The model under review builds one solid part; all positions refer to its coordinate system, in mm. A direction names the side the tool comes from. Give positions to 0.01 mm unless a question says otherwise; leave off trailing zeros. Loops run counter-clockwise (first coordinate to the right, second up) from the corner with the lowest first, then second, coordinate; pieces in that order, holes last. Notation, with made-up numbers: M -37,86 L -5,86 A23 ccw -5,112 Z; hole C 1,12 d9. An arc over 180 degrees is marked long. Write item = value, one per line. Start each with the question number.
1. Draft analysis for pull direction Y (two halves, no side actions). For faces 1 (the face through (8.5, 1.11, 43.65)), 2 (the face through (-6.33, 2.36, 43.65)), 3 (the face through (0, -3.969, 23)), state which applies: pulls with the +Y half, pulls with the -Y half, needs draft (parallel to the pull), parting line crosses it, or undercut.
2. We need section D-D on z = 26.5. Give the boundary of the cut face in (x, y) (3 decimals).
3. For faces 4 (the face through (6.236, -2.417, 43.645)), 5 (the face through (-12.687, -0.496, 4.829)), 6 (the face through (-9.181, -0.714, 43.645)), list the 3-axis set-ups (+Z, -Z, +X, -X, +Y, -Y) from which the entire face can be reached by the end or side of a thin tool; tool diameter is ignored.
4. We need section C-C on z = 39.5. Give the boundary of the cut face in (x, y) (3 decimals), then the cut area to 3 significant figures.
5. We need section B-B on x = 1.5. Give the boundary of the cut face in (y, z), then the cut area to 3 significant figures.
6. We need section A-A on z = 10. Give the boundary of the cut face in (x, y) (1 decimal).
7. Wall thickness on line 1 along Y through (x, z) = (11, 4); line 2 along Z through (x, y) = (-8.5, -1.5); line 3 along Z through (x, y) = (5, -1.75): over which ranges is each line inside the solid? List them lowest first. Write a range as from..to.
8. For pin 1 (4 mm diameter, centred on y = -2, z = 33, fed in from +X) (3 decimals); pin 2 (1 mm diameter, centred on x = -6, z = 10.5, fed in from -Y); pin 3 (3 mm diameter, centred on x = 11.11, y = 0, fed in from -Z); pin 4 (2.5 mm diameter, centred on x = 5.5, y = 1, fed in from +Z), all flat-tipped, find the tip position at first contact; note any pin that passes through.
from build123d import *

# Parameters (mm, degrees)
F0_R     = 7.9375
F0_R_2   = 3.175
F1_DEPTH = 3.96875
F2_R     = 0.79375
F4_D     = 3.302
F4_DEPTH = 9.525
F4_TIP   = 0.992020882
F6_R     = 3.302
F7_DEPTH = 25.4
F9_DEPTH = 1.5875


with BuildPart() as f1:
    # F0 (on Front) → F1 (new body, symmetric)
    with BuildSketch(Plane.XZ):
        with BuildLine():
            Line((-15.875, 7.9375), (-15.875, 0))
            Line((-15.875, 0), (15.875, 0))
            Line((15.875, 0), (15.875, 7.9375))
            Line((15.875, 7.9375), (9.525, 25.4))
            Line((9.525, 25.4), (9.525, 42.8625))
            Line((9.525, 42.8625), (5.9398811015, 42.8625))
            ThreePointArc((5.9398811015, 42.8625), (0, 46.0375), (-5.9398811015, 42.8625))
            Line((-5.9398811015, 42.8625), (-9.525, 42.8625))
            Line((-9.525, 42.8625), (-9.525, 25.4))
            Line((-9.525, 25.4), (-15.875, 7.9375))
        make_face()
        with Locations((0, 12.7)):
            Circle(F0_R, mode=Mode.SUBTRACT)
        with Locations((0, 38.89375)):
            Circle(F0_R_2, mode=Mode.SUBTRACT)
    extrude(amount=F1_DEPTH, both=True)

    # F2
    f2_edges = [f1.edges().sort_by_distance(p)[0] for p in [
        (-9.525, 0, 42.8625),
        (9.525, 0, 42.8625),
    ]]
    fillet(f2_edges, radius=F2_R)

    # F4
    with Locations(Plane(origin=(0, 0, 0), x_dir=(1, 0, 0), z_dir=(0, 0, -1))):
        with Locations((-11.1125, 0), (11.1125, 0)):
            Hole(F4_D / 2, depth=F4_DEPTH)
            with Locations((0, 0, -(F4_DEPTH + F4_TIP / 2))):  # 118° drill point
                Cone(0, F4_D / 2, F4_TIP, mode=Mode.SUBTRACT)

    # F6 (on offset) → F7 (cut)
    with BuildSketch(Plane.XY.offset(42.8625)):
        with Locations((-6.35, 0)):
            Circle(F6_R)
        with Locations((6.35, 0)):
            Circle(F6_R)
    extrude(amount=F7_DEPTH, mode=Mode.SUBTRACT)

    # F8 (on offset) → F9 (join)
    with BuildSketch(Plane.XY.offset(42.8625)):
        Polygon((-4.9855054388, 2.0637681785), (-7.7144945612, 2.6629796349), (-9.5979214659, 0.5992114563), (-8.7523592481, -2.0637681785), (-6.0233701256, -2.6629796349), (-4.139943221, -0.5992114563), align=None)
        Polygon((9.1418760206, -0.1089233026), (7.8402683574, 2.3633739067), (5.0483923368, 2.4722972093), (3.5581239794, 0.1089233026), (4.8597316426, -2.3633739067), (7.6516076632, -2.4722972093), align=None)
    extrude(amount=F9_DEPTH)


solid = f1.part
Final values:
q1.face_1 = pulls with the +Y half
q1.face_2 = undercut
q1.face_3 = pulls with the -Y half
q2.outline = M -9.525,-3.969 L 9.525,-3.969 L 9.525,3.969 L -9.525,3.969 Z
q3.face_4 = +Z
q3.face_5 = -Z
q3.face_6 = +Z, -X, -Y
q4.outline = M -9.525,-3.969 L -3.117,-3.969 L -3.117,3.969 L -9.525,3.969 Z; M 3.117,-3.969 L 9.525,-3.969 L 9.525,3.969 L 3.117,3.969 Z
q4.area = 102 mm²
q5.outline = M -3.97,0 L 3.97,0 L 3.97,4.91 L -3.97,4.91 Z; M -3.97,20.49 L 3.97,20.49 L 3.97,36.1 L -3.97,36.1 Z; M -3.97,41.69 L 3.97,41.69 L 3.97,45.88 L -3.97,45.88 Z
q5.area = 196 mm²
q6.outline = M -15.1,-4 L -7.5,-4 L -7.5,4 L -15.1,4 Z; M 7.5,-4 L 15.1,-4 L 15.1,4 L 7.5,4 Z; hole C -11.1,0 d1.7; hole C 11.1,0 d1.7
q7.line_1 = -3.97..-1.65, 1.65..3.97
q7.line_2 = 0..44.45
q7.line_3 = 0..6.54, 18.86..44.45
q8.pin_1 = 9.525
q8.pin_2 = through
q8.pin_3 = 9.61
q8.pin_4 = 44.45
